Verification items for the finished model (mm, model axes). A direction names the side the tool comes from. Give positions to 0.01 mm unless a question says otherwise; leave off trailing zeros. Order: outer loops, then holes, each group sorted by start corner. A loop starts at its lowest first (then second) coordinate and runs counter-clockwise, first axis right, second up. Notation, with made-up numbers: (0.5, 51.5) -> (34.5, 51.5) arc R28 ccw to (34.5, 71.5) -> close; hole circle Ø10 at (12, 1). An arc over 180 degrees is marked (long way). Return JSON: item names as keys, results as strings. Group by question number.
(1) Cross-section at A-A on z = -25.4. Enter the section's corners in (x, y) (1 decimal).
(2) Thickness scan on line 1 along X through (y, z) = (-6.5, -24); line 2 along Y through (x, z) = (-8, -23) (3 decimals); line 3 along Z through (x, y) = (10.5, -11). Record the ranges inside material, lowest first.
(3) Cross-section at B-B on y = -3.75. Enter the section's corners in (x, z), then the cut area to 3 significant figures.
(4) Cross-section at C-C on x = -5.25. Enter the section's corners in (y, z) (3 decimals).
(5) Tool access check on faces 5 (the face through (10.16, -8, -27)), 6 (the face through (-11, -8, -19.05)), 7 (the face through (-12.7, -2, -15)). Record the directions out of +Z, -Z, +X, -X, +Y, -Y that give a thin tool (end or side, any length) a straight path to the whole face; none if there is none.
(6) Cross-section at D-D on z = 20. Enter the section's corners in (x, y) (3 decimals), then the cut area to 3 significant figures.
(7) Depth check by flat-ended pin: pin 1 Ø3 at (y, z) = (-5.5, -4) entering from +X; pin 2 Ø2 at (x, y) = (-12, -6) entering from +Z; pin 3 Ø5 at (x, z) = (7, -23.5) entering from -Y (3 decimals). Enter the tip coordinate at first touch or a pass-through.
(8) Release check for a two-part mould opening along Z. For faces 1 (the face through (11.41, -7.77, -24.14)), 2 (the face through (11, -8, -19.05)), 3 (the face through (-11.45, -7.77, -24.14)), 4 (the face through (-11, -12.7, -25)) record: pulls with the +Z half, pulls with the -Z half, needs draft (parallel to the pull), parting line crosses it, or undercut.
from build123d import *

# Parameters (mm, degrees)
F1_DEPTH = 3.175
F2_W     = 2.54
F2_H     = 12.7
F3_DEPTH = 12.7
F5_D     = 2.54


with BuildPart() as f1:
    # F0 (on Front) → F1 (new body)
    with BuildSketch(Plane.XZ):
        with BuildLine():
            Line((-12.7, -31.75), (12.7, -31.75))
            Line((12.7, -31.75), (12.7, 25.4))
            ThreePointArc((12.7, 25.4), (10.840128, 29.890128), (6.35, 31.75))
            Line((6.35, 31.75), (-6.35, 31.75))
            ThreePointArc((-6.35, 31.75), (-10.840128, 29.890128), (-12.7, 25.4))
            Line((-12.7, 25.4), (-12.7, -31.75))
        make_face()
    extrude(amount=F1_DEPTH)

    # F2 (on Front) → F3 (join)
    with BuildSketch(Plane.XZ):
        with Locations((11.43, -25.4)):
            Rectangle(F2_W, F2_H)
        with Locations((-11.43, -25.4)):
            Rectangle(F2_W, F2_H)
    extrude(amount=F3_DEPTH)

    # F5 (through all)
    with Locations(Plane.YZ.offset(12.7)):
        with Locations((-7.9375, -25.4)):
            Hole(F5_D / 2)


solid = f1.part
Verdict:
{
 "1": {"outline": "(-12.7, -12.7) -> (-10.2, -12.7) -> (-10.2, -9.2) -> (-12.7, -9.2) -> close; (-12.7, -6.7) -> (-10.2, -6.7) -> (-10.2, -3.2) -> (10.2, -3.2) -> (10.2, -6.7) -> (12.7, -6.7) -> (12.7, 0) -> (-12.7, 0) -> close; (10.2, -12.7) -> (12.7, -12.7) -> (12.7, -9.2) -> (10.2, -9.2) -> close"},
 "2": {"line 1": "-12.7 to -10.16, 10.16 to 12.7", "line 2": "-3.175 to 0", "line 3": "-31.75 to -19.05"},
 "3": {"outline": "(-12.7, -31.75) -> (-10.16, -31.75) -> (-10.16, -19.05) -> (-12.7, -19.05) -> close; (10.16, -31.75) -> (12.7, -31.75) -> (12.7, -19.05) -> (10.16, -19.05) -> close", "area": "64.5 mm²"},
 "4": {"outline": "(-3.175, -31.75) -> (0, -31.75) -> (0, 31.75) -> (-3.175, 31.75) -> close"},
 "5": {"face 5": "+Z, -Z, -Y", "face 6": "+Z, +X, -X, -Y", "face 7": "+Z, -Z, -X, +Y, -Y"},
 "6": {"outline": "(-12.7, -3.175) -> (12.7, -3.175) -> (12.7, 0) -> (-12.7, 0) -> close", "area": "80.6 mm²"},
 "7": {"pin 1": "through", "pin 2": "z = -19.05", "pin 3": "y = -3.175"},
 "8": {"face 1": "undercut", "face 2": "pulls with the +Z half", "face 3": "undercut", "face 4": "needs draft"}
}
